Read the model definition and answer for the solid it produces. Units are mm, in the model's axes. A direction names the side the tool comes from. Give positions to 0.01 mm unless a question says otherwise; leave off trailing zeros. Write each loop counter-clockwise with the first axis right and the second up, starting at its lowest first coordinate (ties: lowest second). Pieces come first, ordered by that corner, then holes. Notation, with made-up numbers: (-37.75, 56) - (-4.75, 56) arc R25 ccw to (-4.75, 95) - close; hole circle Ø2 at (53.25, -38). An arc over 180 degrees is marked (long way). Answer as CSV lines item,"result".
```python
from build123d import *

# Parameters (mm, degrees)
PAD_DEPTH     = 3
POCKET_DEPTH  = 1
SKETCH002_R   = 7.95
SKETCH002_R_2 = 10
SKETCH002_R_3 = 5
PAD001_DEPTH  = 1


with BuildPart() as part:
    # Sketch → Pad (new body)
    with BuildSketch(Plane.XY):
        with BuildLine():
            ThreePointArc((51.681196, 37.715878), (0, 48.9), (-51.681196, 37.715878))
            ThreePointArc((-51.681196, 37.715878), (-59.837802, 31.729345), (-64.898683, 22.968279))
            ThreePointArc((-64.898683, 22.968279), (-71.033558, -11.241914), (-67.511606, -45.818928))
            ThreePointArc((-67.511606, -45.818928), (-60.179833, -52.071942), (-51.92059, -47.108074))
            ThreePointArc((-51.92059, -47.108074), (-46.154899, -30.597197), (-42.75, -13.44322))
            ThreePointArc((-38.952909, -20.742528), (-40.475487, -16.897296), (-42.75, -13.44322))
            ThreePointArc((-38.952909, -20.742528), (-13.396354, -30.88815), (-10.33233, -3.562651))
            ThreePointArc((-15.112075, 3.225883), (-13.051436, -0.400195), (-10.33233, -3.562651))
            ThreePointArc((15.112075, 3.225883), (0, 5), (-15.112075, 3.225883))
            ThreePointArc((10.33233, -3.562652), (13.051436, -0.400195), (15.112075, 3.225883))
            ThreePointArc((10.33233, -3.562652), (13.396355, -30.88815), (38.952909, -20.742528))
            ThreePointArc((42.75, -13.44322), (40.475487, -16.897296), (38.952909, -20.742528))
            ThreePointArc((42.75, -13.44322), (46.154899, -30.597197), (51.92059, -47.108074))
            ThreePointArc((51.92059, -47.108074), (60.179833, -52.071942), (67.511606, -45.818928))
            ThreePointArc((67.511606, -45.818928), (71.033558, -11.241914), (64.898683, 22.968279))
            ThreePointArc((64.898683, 22.968279), (59.837802, 31.729345), (51.681196, 37.715878))
        make_face()
    extrude(amount=PAD_DEPTH)

    # Sketch001 (on Face18 of Pad) → Pocket (cut)
    with BuildSketch(Plane.XY.offset(3)):
        with BuildLine():
            ThreePointArc((-50.027397, 34.07377), (-56.859073, 29.059669), (-61.097882, 21.72172))
            ThreePointArc((-61.097882, 21.72172), (-67.036441, -11.393747), (-63.627191, -44.864296))
            ThreePointArc((-63.627191, -44.864296), (-59.850217, -48.085546), (-55.595456, -45.528402))
            ThreePointArc((-55.595456, -45.528402), (-49.278768, -26.711037), (-46.123539, -7.114141))
            ThreePointArc((-44.554869, -6.371105), (-45.55462, -6.287844), (-46.123539, -7.114141))
            ThreePointArc((-35.102525, -19.658763), (-38.674758, -12.194065), (-44.554869, -6.371105))
            ThreePointArc((-35.102525, -19.658763), (-15.455001, -27.458576), (-13.099421, -6.451112))
            ThreePointArc((-20.008465, 5.014144), (-17.316595, -1.178063), (-13.099421, -6.451112))
            ThreePointArc((-19.325882, 6.248668), (-19.921945, 5.772272), (-20.008465, 5.014144))
            ThreePointArc((19.325882, 6.248667), (0, 9), (-19.325882, 6.248668))
            ThreePointArc((20.008465, 5.014144), (19.921946, 5.772272), (19.325882, 6.248667))
            ThreePointArc((13.099421, -6.451112), (17.316595, -1.178063), (20.008465, 5.014144))
            ThreePointArc((13.099421, -6.451112), (15.455001, -27.458576), (35.102525, -19.658763))
            ThreePointArc((44.554869, -6.371105), (38.674758, -12.194065), (35.102525, -19.658763))
            ThreePointArc((46.123539, -7.114141), (45.55462, -6.287844), (44.554869, -6.371105))
            ThreePointArc((46.123539, -7.114141), (49.278768, -26.711037), (55.595456, -45.528402))
            ThreePointArc((55.595456, -45.528402), (59.850217, -48.085546), (63.627191, -44.864296))
            ThreePointArc((63.627191, -44.864296), (67.036441, -11.393747), (61.097882, 21.72172))
            ThreePointArc((61.097882, 21.72172), (56.859073, 29.059669), (50.027397, 34.07377))
            ThreePointArc((50.027397, 34.07377), (0, 44.9), (-50.027397, 34.07377))
        make_face()
    extrude(amount=-POCKET_DEPTH, mode=Mode.SUBTRACT)

    # Sketch002 (on Face39 of Pocket) → Pad001 (join)
    with BuildSketch(Plane.XY.offset(2)):
        with Locations((41.5, 15.29415)):
            Circle(SKETCH002_R)
        with Locations((-41.5, 15.29415)):
            Circle(SKETCH002_R_2)
        with Locations((27.253882, 7.06915)):
            Circle(SKETCH002_R_3)
        with Locations((22.3, -16.055244)):
            Circle(SKETCH002_R_3)
        with BuildLine():
            ThreePointArc((55.269663, 27.35096), (50.459805, 26.182512), (51.628253, 21.372655))
            ThreePointArc((53.310577, 15.094137), (53.726752, 18.570298), (51.628253, 21.372655))
            ThreePointArc((53.310577, 15.094137), (54.7036, 10.344454), (59.453283, 11.737477))
            ThreePointArc((59.453283, 11.737477), (60.488233, 20.382032), (55.269663, 27.35096))
        make_face()
        with BuildLine():
            ThreePointArc((26.290165, 25.474091), (28.663681, 21.130541), (33.007231, 23.504058))
            ThreePointArc((38.636396, 26.754058), (35.170967, 26.256356), (33.007231, 23.504058))
            ThreePointArc((38.636396, 26.754058), (42.863696, 29.328924), (40.28883, 33.556224))
            ThreePointArc((40.28883, 33.556224), (31.670967, 32.318534), (26.290165, 25.474091))
        make_face()
        Polygon((-25.05, -13.305244), (-25.05, -7.305244), (-19.55, -7.305244), (-19.55, -13.305244), (-13.55, -13.305244), (-13.55, -18.805244), (-19.55, -18.805244), (-19.55, -24.805244), (-25.05, -24.805244), (-25.05, -18.805244), (-31.05, -18.805244), (-31.05, -13.305244), align=None)
    extrude(amount=PAD001_DEPTH)


solid = part.part
```
(1) A cutting plane is placed at A-A (z = 0.8). Write down the section's boundary in (x, y) (3 decimals).
Worked out:
outline,"(-67.512, -45.819) arc R8.25 ccw to (-51.921, -47.108) arc R125 ccw to (-42.75, -13.443) arc R20.18 cw to (-38.953, -20.743) arc R17.3 ccw (long way) to (-10.332, -3.563) arc R21.6 cw to (-15.112, 3.226) arc R65.25 cw to (15.112, 3.226) arc R21.6 cw to (10.332, -3.563) arc R17.3 ccw (long way) to (38.953, -20.743) arc R20.18 cw to (42.75, -13.443) arc R125 ccw to (51.921, -47.108) arc R8.25 ccw to (67.512, -45.819) arc R125 ccw to (64.899, 22.968) arc R24.625 ccw to (51.681, 37.716) arc R125 ccw to (-51.681, 37.716) arc R24.625 ccw to (-64.899, 22.968) arc R125 ccw to start"
(2) Each of these flat-tipped pins is pushed along its axis until it touches: P1, Ø0.5, axis at x = -28.5, z = 2.5, coming from the -Y side; P2, Ø5, axis at x = -32, y = -32, coming from the +Z side; P3, Ø1.1, axis at y = -11.5, z = 2.5, coming from the -X side; P4, Ø1.1, axis at x = -21.5, z = 2.5, coming from the -Y side. Where does it stop, or does it pass through?
Worked out:
P1,"stops at y = -32.3"
P2,"stops at z = 3"
P3,"stops at x = -71.06"
P4,"stops at y = -33.35"
(3) Find the intervals of material crossed by L1, parallel to X at y = -42.5, z = 2.7; L2, parallel to Y at x = -22.3, z = 2.4; L3, parallel to Z at x = -50, y = -29, in increasing order.
Worked out:
L1,"x = -68.28 to -64.18, -54.34 to -50.05, 50.05 to 54.34, 64.18 to 68.28"
L2,"y = -33.36 to -29.36, -24.81 to -7.31, 42.83 to 46.89"
L3,"z = 0 to 2"
(4) For faces 4 (the cylindrical face through (31.78, 32.38, 2.49)), 5 (the flat face through (-42, 15, 3)), determine the directions among +Z, -Z, +X, -X, +Y, -Y from which every point of the face is accessible in a straight line to the end or side of a thin tool.
Worked out:
face 4,"+Z"
face 5,"+Z, +X, -X, +Y, -Y"
(5) A cutting plane is placed at C-C (y = 42.5). Write down the section's boundary in (x, z).
Worked out:
outline,"(-39.48, 0) - (39.48, 0) - (39.48, 3) - (23.98, 3) - (23.98, 2) - (-23.98, 2) - (-23.98, 3) - (-39.48, 3) - close"
(6) A cutting plane is placed at D-D (x = -59). Write down the section's boundary in (y, z).
Worked out:
outline,"(-52.08, 0) - (32.62, 0) - (32.62, 3) - (26.21, 3) - (26.21, 2) - (-48.07, 2) - (-48.07, 3) - (-52.08, 3) - close"
(7) The mould has two halves that part along Y. Classify faces 1 (the cylindrical face through (-60.32, -52.06, 1.48)), 2 (the cylindrical face through (42.845, 29.254, 2.493)), 3 (the flat face through (27, 7, 3)): +Y half, -Y half, draft (parallel to the pull), parting line (faces both ways), or undercut.
Worked out:
face 1,"-Y half"
face 2,"undercut"
face 3,"draft"
(8) A cutting plane is placed at B-B (x = -22.3). Write down the section's boundary in (y, z), and give its area (3 significant figures).
Worked out:
outline,"(-33.36, 0) - (46.89, 0) - (46.89, 3) - (42.83, 3) - (42.83, 2) - (-7.31, 2) - (-7.31, 3) - (-24.81, 3) - (-24.81, 2) - (-29.36, 2) - (-29.36, 3) - (-33.36, 3) - close"
area,"186 mm^2"
